```python
from build123d import *

# Parameters (mm, degrees)
F0_W     = 50.8
F0_H     = 53.975
F0_R     = 2.5527
F1_DEPTH = 3.175
F2_W     = 50.8
F2_H     = 3.175
F3_DEPTH = 50.8
F4_R     = 2.5527
F5_DEPTH = 25.4


with BuildPart() as f1:
    # F0 (on Top) → F1 (new body)
    with BuildSketch(Plane.XY):
        with Locations((25.4, -26.9875)):
            Rectangle(F0_W, F0_H)
        with Locations((12.7, -28.575)):
            Circle(F0_R, mode=Mode.SUBTRACT)
        with Locations((38.1, -28.575)):
            Circle(F0_R, mode=Mode.SUBTRACT)
    extrude(amount=F1_DEPTH)

    # F2 (on face) → F3 (join)
    with BuildSketch(Plane.XY.offset(3.175)):
        with Locations((25.4, -1.5875)):
            Rectangle(F2_W, F2_H)
    extrude(amount=F3_DEPTH)

    # F4 (on face) → F5 (cut)
    with BuildSketch(Plane.XZ.offset(3.175)):
        with Locations((12.7, 28.575)):
            Circle(F4_R)
        with Locations((38.1, 28.575)):
            Circle(F4_R)
    extrude(amount=-F5_DEPTH, mode=Mode.SUBTRACT)


solid = f1.part
```
Geometry: final body of the model. Coordinates: model frame, mm. A direction names the side the tool comes from. Round coordinates to 2 decimals unless told otherwise and drop trailing zeros. Order: outer loops, then holes, each group sorted by start corner. A loop starts at its lowest first (then second) coordinate and runs counter-clockwise, first axis right, second up. Notation, with made-up numbers: (26, 62) -> (68, 62) arc R12 cw to (68, 82) -> close; hole circle Ø7 at (-3.5, 15). An arc over 180 degrees is marked (long way). Use one line per item in the form item = value. Start each with the question number.
1. Cut plane A-A (x = 38.1). Return the cut outline in (y, z) (3 decimals).
2. Reachability of faces 4 (the face through (37.547, -31.067, 1.565)), 5 (the face through (25, -3.175, 28)) from +Z, -Z, +X, -X, +Y, -Y: full face, straight path, thin tool, end or side. Return the list, or none.
3. Cut plane C-C (x = 25.5). Return the cut outline in (y, z) (3 decimals), then the cut area to 3 significant figures.
4. Draft query along Z for faces 1 (the face through (25, 0, 27)), 2 (the face through (14.07, -1.61, 30.73)), 3 (the face through (25, -28, 3.175)). Return one class per face: pulls with the +Z half, pulls with the -Z half, needs draft (parallel to the pull), parting line crosses it, or undercut.
5. Pin query (flat end, axial travel): pin 1 Ø15 at (x, z) = (19, 21) entering from -Y (3 decimals); pin 2 Ø1.5 at (x, y) = (20.5, -28.5) entering from +Z (3 decimals). Return the tip coordinate at first contact, or that it passes through.
6. Cut plane B-B (y = -27). Return the cut outline in (x, z) (3 decimals).
7. Cut plane D-D (z = 23.5). Return the cut outline in (x, y) (3 decimals), then the cut area to 3 significant figures.
8. Line query: probe 1 along Z at (x, y) = (12.7, -2.4) (3 decimals); probe 2 along Y at (x, z) = (12.7, 0.95) (3 decimals); probe 3 along Y at (x, z) = (2.5, 23.5) (3 decimals). Output: solid intervals per line, ascending.
Solution:
q1.outline = (-53.975, 0) -> (-31.128, 0) -> (-31.128, 3.175) -> (-53.975, 3.175) -> close; (-26.022, 0) -> (0, 0) -> (0, 26.022) -> (-3.175, 26.022) -> (-3.175, 3.175) -> (-26.022, 3.175) -> close; (-3.175, 31.128) -> (0, 31.128) -> (0, 53.975) -> (-3.175, 53.975) -> close
q2.face_4 = +Z, -Z
q2.face_5 = +Z, +X, -X, -Y
q3.outline = (-53.975, 0) -> (0, 0) -> (0, 53.975) -> (-3.175, 53.975) -> (-3.175, 3.175) -> (-53.975, 3.175) -> close
q3.area = 333 mm^2
q4.face_1 = needs draft
q4.face_2 = undercut
q4.face_3 = pulls with the +Z half
q5.pin_1 = -3.175
q5.pin_2 = 3.175
q6.outline = (0, 0) -> (10.691, 0) -> (10.691, 3.175) -> (0, 3.175) -> close; (14.709, 0) -> (36.091, 0) -> (36.091, 3.175) -> (14.709, 3.175) -> close; (40.109, 0) -> (50.8, 0) -> (50.8, 3.175) -> (40.109, 3.175) -> close
q7.outline = (0, -3.175) -> (50.8, -3.175) -> (50.8, 0) -> (0, 0) -> close
q7.area = 161 mm^2
q8.probe_1 = 0 to 26.022, 31.128 to 53.975
q8.probe_2 = -53.975 to -31.128, -26.022 to 0
q8.probe_3 = -3.175 to 0
